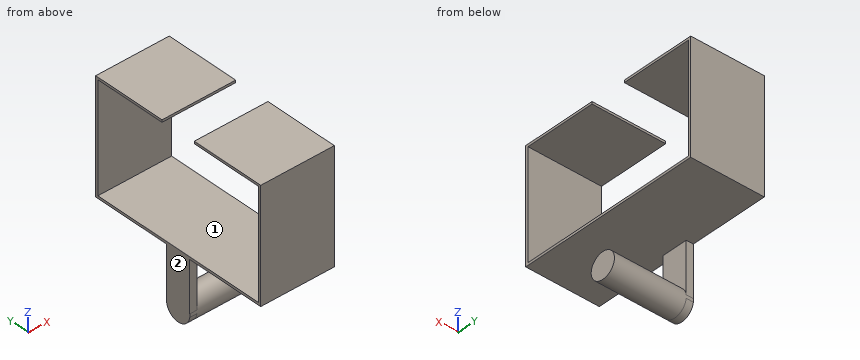
from build123d import *

# Parameters (mm, degrees)
BOSS_EXTRUDE1_DEPTH = 26.04516
BOSS_EXTRUDE2_DEPTH = 2.54
SKETCH5_R           = 4.572
BOSS_EXTRUDE3_DEPTH = 27.94


with BuildPart() as part:
    # Sketch1 → Boss-Extrude1 (new body)
    with BuildSketch(Plane.YZ):
        Polygon((-32.39516, 0), (32.39516, 0), (32.39516, 39.7764), (6.3246, 39.7764), (6.3246, 38.94836), (31.5214, 38.94836), (31.5214, 0.87376), (-31.5214, 0.87376), (-31.5214, 38.94836), (-6.3246, 38.94836), (-6.3246, 39.7764), (-32.39516, 39.7764), align=None)
    extrude(amount=BOSS_EXTRUDE1_DEPTH)

    # Sketch2 → Boss-Extrude2 (add)
    with BuildSketch(Plane.YZ):
        with BuildLine():
            Line((-4.5339, 0), (4.5339, 0))
            Line((4.5339, 0), (4.5339, -19.05))
            ThreePointArc((4.5339, -19.05), (0, -23.032988294), (-4.5339, -19.05))
            Line((-4.5339, -19.05), (-4.5339, 0))
        make_face()
    extrude(amount=BOSS_EXTRUDE2_DEPTH)

    # Sketch5 → Boss-Extrude3 (add)
    with BuildSketch(Plane.YZ):
        with Locations(Location((0, -18.460988294, 0), (0, 0, 7.401999688))):
            Circle(SKETCH5_R)
    extrude(amount=BOSS_EXTRUDE3_DEPTH)


solid = part.part
The listing builds one solid part. Answer for the finished solid, in the listing's coordinates (mm). Face numbers are marked on the shaded views. A direction names the side the tool comes from. Give positions to 0.01 mm unless a question says otherwise; leave off trailing zeros. Write each loop counter-clockwise with the first axis right and the second up, starting at its lowest first coordinate (ties: lowest second). Pieces come first, ordered by that corner, then holes. Notation, with made-up numbers: (46.5, 66.25) - (79.5, 66.25) arc R16 cw to (79.5, 96.25) - close; hole circle Ø7 at (-4.5, 27.5). An arc over 180 degrees is marked (long way). One line per question, with ' | ' between items. Start each with the question number.
1. Section C-C, the plane z = 32 is taken. Determine the outline of the cut face in (x, y), then the cut area to 3 significant figures.
2. Section B-B, the plane y = -12.5 is taken. Determine the outline of the cut face in (x, z), then the cut area to 3 significant figures.
3. Given P1, Ø4.5, axis at y = 0, z = -6.5, coming from the +X side; P2, Ø20, axis at y = -16, z = 13, coming from the +X side; P3, Ø7.5, axis at x = 9.5, y = -22.5, coming from the -Z side; P4, Ø0.8, axis at x = 1, z = -11.5, coming from the +Y side, each flat-ended and moving along its own axis, determine where each tip first touches the part or whether it passes through.
4. For the marked faces 1 and 2, determine the directions among +Z, -Z, +X, -X, +Y, -Y from which every point of the face is accessible in a straight line to the end or side of a thin tool.
5. Straight lines are drawn through the part: line 1 (Y direction, x = 9.75, z = 35.5); line 2 (Z direction, x = 22, y = -19); line 3 (Z direction, x = 17.5, y = 5). For each, find the intervals that lie inside material, in ascending order.
6. Section A-A, the plane x = 19 is taken. Determine the outline of the cut face in (y, z), then the cut area to 3 significant figures.
7. Section D-D, the plane y = 0 is taken. Determine the outline of the cut face in (x, z), then the cut area to 3 significant figures.
Result:
1) outline: (0, -32.4) - (26.05, -32.4) - (26.05, -31.52) - (0, -31.52) - close; (0, 31.52) - (26.05, 31.52) - (26.05, 32.4) - (0, 32.4) - close | area: 45.5 mm2
2) outline: (0, 0) - (26.05, 0) - (26.05, 0.87) - (0, 0.87) - close; (0, 38.95) - (26.05, 38.95) - (26.05, 39.78) - (0, 39.78) - close | area: 44.3 mm2
3) P1: stops at x = 2.54 | P2: passes through | P3: stops at z = 0 | P4: stops at y = 4.53
4) face 1: +X, -X | face 2: +Z, -Z, -X, +Y, -Y
5) line 1: y = -32.4 to -31.52, 31.52 to 32.4 | line 2: z = 0 to 0.87, 38.95 to 39.78 | line 3: z = 0 to 0.87
6) outline: (-32.4, 0) - (32.4, 0) - (32.4, 39.78) - (6.32, 39.78) - (6.32, 38.95) - (31.52, 38.95) - (31.52, 0.87) - (-31.52, 0.87) - (-31.52, 38.95) - (-6.32, 38.95) - (-6.32, 39.78) - (-32.4, 39.78) - close; circle Ø9.14 at (0, -18.46) | area: 232 mm2
7) outline: (0, -23.03) - (27.94, -23.03) - (27.94, -13.89) - (2.54, -13.89) - (2.54, 0) - (26.05, 0) - (26.05, 0.87) - (0, 0.87) - close | area: 314 mm2
